```python
from build123d import *

# Parameters (mm, degrees)
SKETCH2_W           = 38.1
SKETCH2_H           = 381
SKETCH2_R           = 5.08
SKETCH2_R_2         = 4.7625
BOSS_EXTRUDE2_DEPTH = 4.7625


with BuildPart() as part:
    # Sketch2 → Boss-Extrude2 (new body)
    with BuildSketch(Plane.XY):
        with Locations((19.05, 190.5)):
            Rectangle(SKETCH2_W, SKETCH2_H)
        with Locations(Location((11.43, 78.69046619, 0), (0, 0, 180))):
            Circle(SKETCH2_R, mode=Mode.SUBTRACT)
        with Locations(Location((26.67, 73.61046619, 0), (0, 0, 180))):
            Circle(SKETCH2_R, mode=Mode.SUBTRACT)
        with Locations(Location((6.985, 12.01546619, 0), (0, 0, 180))):
            Circle(SKETCH2_R, mode=Mode.SUBTRACT)
        with Locations(Location((29.21, 19.00046619, 0), (0, 0, 180))):
            Circle(SKETCH2_R, mode=Mode.SUBTRACT)
        with Locations(Location((19.05, 114.3, 0), (0, 0, 180))):
            Circle(SKETCH2_R_2, mode=Mode.SUBTRACT)
        with Locations(Location((19.05, 189.23, 0), (0, 0, 180))):
            Circle(SKETCH2_R_2, mode=Mode.SUBTRACT)
    extrude(amount=BOSS_EXTRUDE2_DEPTH)


solid = part.part
```
Design review of the part built by this model. Coordinates are the model's own, in mm. Give positions to 0.01 mm unless a question says otherwise; leave off trailing zeros. Order: outer loops, then holes, each group sorted by start corner. A loop starts at its lowest first (then second) coordinate and runs counter-clockwise, first axis right, second up. Notation, with made-up numbers: (49, 79) -> (90, 79) arc R3 ccw to (90, 83) -> close; hole circle Ø9 at (-12.75, 40.5). An arc over 180 degrees is marked (long way). Write each question's results on one line, items separated by ' | '. Start each with the question number.
Q1. Mouldability with a two-part tool opening along X and no side actions: class faces 1 (the flat face through (23, 193, 4.762)), 2 (the cylindrical face through (33.24, 22.09, 2.35)) as +X half, -X half, draft (parallel to the pull), parting line (faces both ways), or undercut.
Q2. Wall thickness on L1, parallel to Y at x = 8, z = 3.1; L2, parallel to Y at x = 26.67, z = 1.8; L3, parallel to X at y = 114.3, z = 3.85: over which ranges is each line inside the solid? List them lowest first. Write a range as from..to.
Q3. Add section A-A on y = 189.23. Give the boundary of the cut face in (x, z), and give its area (3 significant figures).
Q4. Add section B-B on z = 2.3. State how many separate pieces and enclosed holes the cut face has, and give its area (3 significant figures).
Found:
1) face 1: draft | face 2: undercut
2) L1: y = 0..7.04, 16.99..74.94, 82.44..381 | L2: y = 0..14.6, 23.4..68.53, 78.69..381 | L3: x = 0..14.29, 23.81..38.1
3) outline: (0, 0) -> (14.29, 0) -> (14.29, 4.76) -> (0, 4.76) -> close; (23.81, 0) -> (38.1, 0) -> (38.1, 4.76) -> (23.81, 4.76) -> close | area: 136 mm2
4) separate pieces: 1 | enclosed holes: 6 | area: 14,000 mm2
